Verification items for the finished model (mm, model axes). Face numbers are marked on the shaded views. A direction names the side the tool comes from. Round coordinates to 2 decimals unless told otherwise and drop trailing zeros. Order: outer loops, then holes, each group sorted by start corner. A loop starts at its lowest first (then second) coordinate and runs counter-clockwise, first axis right, second up. Notation, with made-up numbers: (40.5, 73.5) -> (71.5, 73.5) arc R27 cw to (71.5, 112.5) -> close; hole circle Ø5 at (69, -20). An arc over 180 degrees is marked (long way). Return JSON: item names as keys, results as strings. Group by question number.
1) Draft check along X on the marked faces 4, 5, 6 and 7. Enter one of: pulls with the +X half, pulls with the -X half, needs draft (parallel to the pull), parting line crosses it, or undercut.
2) Section check B-B on z = 18.5. Enter the section's corners in (x, y).
3) Section check C-C on x = -11. Enter the section's corners in (y, z), plus the area to 3 significant figures.
4) Scan lines: L1, parallel to X at y = 12.5, z = -7.5; L2, parallel to X at y = 5.5, z = -19.5; L3, parallel to Y at x = 13.3, z = 18.5. Record each from-to range of solid material in increasing order.
5) Section check D-D on y = -13. Enter the section's corners in (x, z), plus the area to 3 significant figures.
6) Tool access check on the marked faces 1, 2 and 3. Record the directions out of +Z, -Z, +X, -X, +Y, -Y that give a thin tool (end or side, any length) a straight path to the whole face; none if there is none.
7) Section check A-A on y = 6. Enter the section's corners in (x, z).
8) Depth check by flat-ended pin: pin 1 (2 mm diameter, centred on y = 12, z = -7.5, fed in from +X); pin 2 (12 mm diameter, centred on x = -11.5, z = 0.5, fed in from -Y); pin 3 (5 mm diameter, centred on x = -3, y = 7.5, fed in from -Z); pin 4 (9.5 mm diameter, centred on y = 1.5, z = 18, fed in from +X). Enter the tip coordinate at first touch or a pass-through.
```python
from build123d import *

# Parameters (mm, degrees)
SKETCH_1_W           = 34
SKETCH_1_H           = 49
EXTRUDE_1_DEPTH      = 10
SKETCH_2_W           = 1.5
SKETCH_2_H           = 24
EXTRUDE_2_DEPTH      = 4
SKETCH_3_W           = 1.5
SKETCH_3_H           = 12
SKETCH_3_W_2         = 25
SKETCH_3_H_2         = 13
CUT_EXTRUDE_1_DEPTH  = 10
SKETCH_4_R           = 2
CUT_EXTRUDE_2_DEPTH  = 31
EXTRUDE_3_DEPTH      = 8
CUT_EXTRUDE_4_DEPTH  = 10
EXTRUDE_4_DEPTH      = 3
EXTRUDE_5_DEPTH      = 3
EXTRUDE_6_DEPTH      = 3
EXTRUDE_7_DEPTH      = 34
EXTRUDE_8_DEPTH      = 3
EXTRUDE_9_REACH      = 31.5
CUT_EXTRUDE_10_DEPTH = 1.5
CUT_EXTRUDE_11_DEPTH = 1.5
CUT_EXTRUDE_12_DEPTH = 25
SKETCH_18_W          = 75
SKETCH_18_H          = 70
SKETCH_18_R          = 1.65
EXTRUDE_10_DEPTH     = 2


with BuildPart() as part:
    # Sketch 1 → Extrude 1 (new body)
    with BuildSketch(Plane(origin=(0, 0, 0), x_dir=(1, 0, 0), z_dir=(0, 1, 0))):
        Rectangle(SKETCH_1_W, SKETCH_1_H)
    extrude(amount=EXTRUDE_1_DEPTH)

    # Sketch 2 → Extrude 2 (add)
    with BuildSketch(Plane(origin=(0, 10, 0), x_dir=(1, 0, 0), z_dir=(0, 1, 0))):
        with Locations((-16.25, 7.5)):
            Rectangle(SKETCH_2_W, SKETCH_2_H)
        with Locations((16.25, 7.5)):
            Rectangle(SKETCH_2_W, SKETCH_2_H)
    extrude(amount=EXTRUDE_2_DEPTH)

    # Sketch 3 → Cut-Extrude 1 (cut)
    with BuildSketch(Plane(origin=(0, 10, 0), x_dir=(1, 0, 0), z_dir=(0, 1, 0))):
        with Locations((-16.25, -18.5)):
            Rectangle(SKETCH_3_W, SKETCH_3_H)
        with Locations((16.25, -18.5)):
            Rectangle(SKETCH_3_W, SKETCH_3_H)
        with Locations((0, -18)):
            Rectangle(SKETCH_3_W_2, SKETCH_3_H_2)
    extrude(amount=-CUT_EXTRUDE_1_DEPTH, mode=Mode.SUBTRACT)

    # Sketch 4 → Cut-Extrude 2 (cut)
    with BuildSketch(Plane.ZY.offset(15.5)):
        with Locations((18.5, 6)):
            Circle(SKETCH_4_R)
    extrude(amount=-CUT_EXTRUDE_2_DEPTH, mode=Mode.SUBTRACT)

    # Sketch 5 → Extrude 3 (add)
    with BuildSketch(Plane.XZ):
        Polygon((4, 11.5), (-4, 11.5), (-4, 41.5), (-13, 41.5), (-13, 56.5), (13, 56.5), (13, 41.5), (4, 41.5), align=None)
    extrude(amount=-EXTRUDE_3_DEPTH)

    # Sketch 5_2 → Cut-Extrude 4 (cut)
    with BuildSketch(Plane.XZ):
        Polygon((4, 11.5), (-4, 11.5), (-4, 41.5), (-13, 41.5), (-13, 56.5), (13, 56.5), (13, 41.5), (4, 41.5), align=None)
    extrude(amount=-CUT_EXTRUDE_4_DEPTH, mode=Mode.SUBTRACT)

    # Sketch 7 → Extrude 4 (add)
    with BuildSketch(Plane.ZY.offset(15.5)):
        Polygon((24.5, 10), (27.713938048, 1.169777784), (24.5, 0), align=None)
    extrude(amount=-EXTRUDE_4_DEPTH)

    # Sketch 8 → Extrude 5 (add)
    with BuildSketch(Plane(origin=(15.5, 0, 0), x_dir=(0, 0, -1), z_dir=(1, 0, 0))):
        Polygon((-27.713938048, 1.169777784), (-24.5, 0), (-24.5, 10), align=None)
    extrude(amount=-EXTRUDE_5_DEPTH)

    # Sketch 9 → Extrude 6 (add)
    with BuildSketch(Plane(origin=(15.5, 0, 0), x_dir=(0, 0, -1), z_dir=(1, 0, 0))):
        Polygon((-12.5, 0), (-24.5, 0), (-13.903733341, -3.856725658), align=None)
    extrude(amount=-EXTRUDE_6_DEPTH)

    # Sketch 10 → Extrude 7 (add)
    with BuildSketch(Plane(origin=(17, 0, 0), x_dir=(0, 0, -1), z_dir=(1, 0, 0))):
        Polygon((-12.5, 0), (-13.903733341, -3.856725658), (18.768088856, -15.748296437), (24.5, 0), align=None)
    extrude(amount=-EXTRUDE_7_DEPTH)

    # Sketch 11 → Extrude 8 (add)
    with BuildSketch(Plane.ZY.offset(15.5)):
        Polygon((24.5, 0), (13.903733341, -3.856725658), (12.5, 0), align=None)
    extrude(amount=-EXTRUDE_8_DEPTH)

    # Sketch 12 → Extrude 9 (add, up to next)
    with BuildSketch(Plane(origin=(-12.5, 0, 0), x_dir=(0, 0, -1), z_dir=(1, 0, 0)), mode=Mode.PRIVATE) as extrude_9_sk1:
        Polygon((-12.5, 0), (-11.5, 2.747477419), (-11.5, 0), align=None)
    extrude_9_tool1 = extrude(extrude_9_sk1.sketch, amount=EXTRUDE_9_REACH, mode=Mode.PRIVATE) - part.part
    add(extrude_9_tool1.solids().sort_by_distance((-12.5, 0.915826, 11.833333))[0])

    # Sketch 13 → Cut-Extrude 10 (cut)
    with BuildSketch(Plane(origin=(17, 0, 0), x_dir=(0, 0, -1), z_dir=(1, 0, 0))):
        Polygon((-12.5, 0), (-8.860297657, 10), (-12.5, 10), align=None)
    extrude(amount=-CUT_EXTRUDE_10_DEPTH, mode=Mode.SUBTRACT)

    # Sketch 16 → Cut-Extrude 11 (cut)
    with BuildSketch(Plane.ZY.offset(17)):
        Polygon((12.5, 10), (12.5, 0), (8.860297657, 10), align=None)
    extrude(amount=-CUT_EXTRUDE_11_DEPTH, mode=Mode.SUBTRACT)

    # Sketch 17 → Cut-Extrude 12 (cut)
    with BuildSketch(Plane(origin=(-12.5, 0, 0), x_dir=(0, 0, -1), z_dir=(1, 0, 0))):
        Polygon((-11.5, 2.747477419), (-11.5, 10), (-8.860297657, 10), align=None)
    extrude(amount=CUT_EXTRUDE_12_DEPTH, mode=Mode.SUBTRACT)

    # Sketch 18 → Extrude 10 (add, symmetric)
    with BuildSketch(Plane(origin=(0, -7.874148219, 2.865955572), x_dir=(1, 0, 0), z_dir=(0, -0.939692621, 0.342020143))):
        with Locations((0, -8.557329357)):
            Rectangle(SKETCH_18_W, SKETCH_18_H)
        with Locations((28.5, 4.942670643)):
            Circle(SKETCH_18_R, mode=Mode.SUBTRACT)
        with Locations((28.5, -35.057329357)):
            Circle(SKETCH_18_R, mode=Mode.SUBTRACT)
        with Locations((-28.5, 4.942670643)):
            Circle(SKETCH_18_R, mode=Mode.SUBTRACT)
        with Locations((-28.5, -35.057329357)):
            Circle(SKETCH_18_R, mode=Mode.SUBTRACT)
    extrude(amount=EXTRUDE_10_DEPTH, both=True)


solid = part.part
```
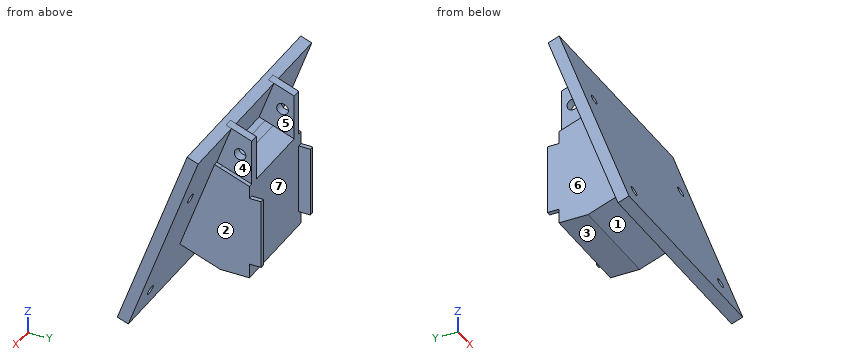
Check result:
{
 "1": {"face 4": "pulls with the +X half", "face 5": "undercut", "face 6": "pulls with the -X half", "face 7": "undercut"},
 "2": {"outline": "(-37.5, -4.31) -> (37.5, -4.31) -> (37.5, -0.06) -> (15.5, -0.06) -> (15.5, 4) -> (12.5, 4) -> (12.5, -0.06) -> (-12.5, -0.06) -> (-12.5, 4) -> (-15.5, 4) -> (-15.5, -0.06) -> (-37.5, -0.06) -> close; (-15.5, 8) -> (-12.5, 8) -> (-12.5, 10) -> (-15.5, 10) -> close; (12.5, 8) -> (15.5, 8) -> (15.5, 10) -> (12.5, 10) -> close"},
 "3": {"outline": "(-24.65, -37.38) -> (-20.89, -38.75) -> (-13.87, -19.45) -> (0, -24.5) -> (10, -24.5) -> (10, 8.86) -> (-1.98, 13.22) -> (3.05, 27.03) -> (-0.71, 28.4) -> close", "area": "925 mm^2"},
 "4": {"L1": "-17 to -15.5, 15.5 to 17", "L2": "-17 to 17", "L3": "-4.31 to 4, 8 to 10"},
 "5": {"outline": "(-37.5, -17.06) -> (-17, -17.06) -> (-17, -19.77) -> (17, -19.77) -> (17, -17.06) -> (37.5, -17.06) -> (37.5, -5.37) -> (-37.5, -5.37) -> close", "area": "969 mm^2"},
 "6": {"face 1": "-Z, +X, -X", "face 2": "-Z, +X, +Y", "face 3": "-Z, +X, -X, +Y"},
 "7": {"outline": "(-17, -24.5) -> (17, -24.5) -> (17, 10.32) -> (15.5, 10.32) -> (15.5, 16.5) -> (12.5, 16.5) -> (12.5, 10.32) -> (-12.5, 10.32) -> (-12.5, 16.5) -> (-15.5, 16.5) -> (-15.5, 10.32) -> (-17, 10.32) -> close; (-15.5, 20.5) -> (-12.5, 20.5) -> (-12.5, 25.96) -> (-15.5, 25.96) -> close; (12.5, 20.5) -> (15.5, 20.5) -> (15.5, 25.96) -> (12.5, 25.96) -> close"},
 "8": {"pin 1": "x = 17", "pin 2": "y = -13.05", "pin 3": "z = -24.5", "pin 4": "x = 37.5"}
}
